The model under review builds one solid part; all positions refer to its coordinate system, in mm. Coordinates: 2 decimals unless noted, no trailing zeros. Order: outer loops, then holes, each group sorted by start corner. A loop starts at its lowest first (then second) coordinate and runs counter-clockwise, first axis right, second up. Notation, with made-up numbers: (49.25, 24) - (86.25, 24) arc R32 ccw to (86.25, 53) - close; hole circle Ø3 at (-35.75, 57). An arc over 180 degrees is marked (long way). Answer in a Markdown table with one row per item.
```python
from build123d import *

# Parameters (mm, degrees)
SKETCH1_W           = 863.6
SKETCH1_H           = 457.2
BOSS_EXTRUDE1_DEPTH = 3.175
SKETCH2_R           = 38.1
SKETCH2_R_2         = 22.225
CUT_EXTRUDE1_DEPTH  = 489.589071332


with BuildPart() as part:
    # Sketch1 → Boss-Extrude1 (new body)
    with BuildSketch(Plane.XY):
        Rectangle(SKETCH1_W, SKETCH1_H)
    extrude(amount=BOSS_EXTRUDE1_DEPTH)

    # Sketch2 → Cut-Extrude1 (cut, through all)
    with BuildSketch(Plane.XY.offset(3.175)):
        with Locations((230.738100004, 0)):
            Circle(SKETCH2_R)
        with Locations((230.738100004, -139.7)):
            Circle(SKETCH2_R)
        with Locations((179.938100004, -67.222799997)):
            Circle(SKETCH2_R_2)
        with Locations((281.538100004, -67.222799997)):
            Circle(SKETCH2_R_2)
        with Locations((179.938100004, 72.477200003)):
            Circle(SKETCH2_R_2)
        with Locations((281.538100004, 72.477200003)):
            Circle(SKETCH2_R_2)
        with Locations((-40.855899988, 120.65)):
            Circle(SKETCH2_R)
    extrude(amount=-CUT_EXTRUDE1_DEPTH, mode=Mode.SUBTRACT)


solid = part.part
```
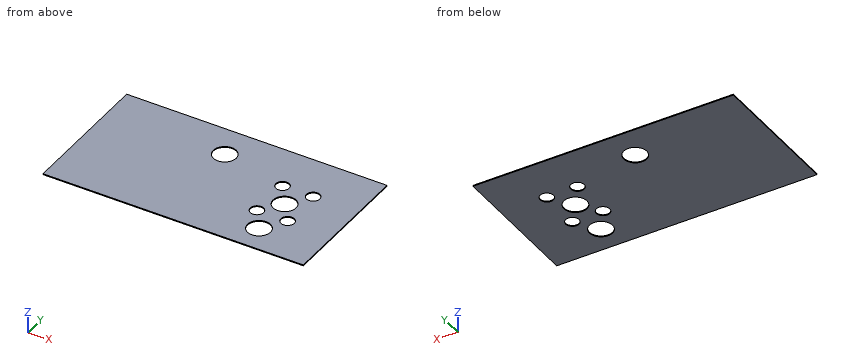
Item 1: Clearance check with a flat-ended pin moving along its axis: pin 1 Ø1.5 at (x, y) = (96, -13) entering from -Z. State where the tip first meets the part, or that it passes through.
Check values:
| item | result |
|---|---|
| pin 1 | z = 0 |
Item 2: We need section C-C, the plane z = 1.4. Write out the cut boundary in (x, y) (3 decimals), then the cut area to 3 significant figures.
Check values:
| item | result |
|---|---|
| outline | (-431.8, -228.6) - (431.8, -228.6) - (431.8, 228.6) - (-431.8, 228.6) - close; hole circle Ø76.2 at (-40.856, 120.65); hole circle Ø44.45 at (179.938, -67.223); hole circle Ø44.45 at (179.938, 72.477); hole circle Ø76.2 at (230.738, -139.7); hole circle Ø76.2 at (230.738, 0); hole circle Ø44.45 at (281.538, -67.223); hole circle Ø44.45 at (281.538, 72.477) |
| area | 375,000 mm^2 |
Item 3: We need section D-D, the plane y = 108. Write out the cut boundary in (x, z) (3 decimals).
Check values:
| item | result |
|---|---|
| outline | (-431.8, 0) - (-76.795, 0) - (-76.795, 3.175) - (-431.8, 3.175) - close; (-4.917, 0) - (431.8, 0) - (431.8, 3.175) - (-4.917, 3.175) - close |
Item 4: To check wall thickness, follow line 1 (X direction, y = -53.5, z = 1.7); line 2 (X direction, y = 92, z = 0.85); line 3 (X direction, y = 112.5, z = 0.8). State the ranges of each line that lie inside material, in increasing order. Write a range as from..to.
Check values:
| item | result |
|---|---|
| line 1 | -431.8..162.46, 197.42..264.06, 299.02..431.8 |
| line 2 | -431.8..-65.97, -15.74..169.32, 190.56..270.92, 292.16..431.8 |
| line 3 | -431.8..-78.07, -3.64..431.8 |
Item 5: We need section A-A, the plane y = -139.7. Write out the cut boundary in (x, z) (3 decimals).
Check values:
| item | result |
|---|---|
| outline | (-431.8, 0) - (192.638, 0) - (192.638, 3.175) - (-431.8, 3.175) - close; (268.838, 0) - (431.8, 0) - (431.8, 3.175) - (268.838, 3.175) - close |
Item 6: We need section B-B, the plane x = 215. Write out the cut boundary in (y, z) (3 decimals).
Check values:
| item | result |
|---|---|
| outline | (-228.6, 0) - (-174.398, 0) - (-174.398, 3.175) - (-228.6, 3.175) - close; (-105.002, 0) - (-34.698, 0) - (-34.698, 3.175) - (-105.002, 3.175) - close; (34.698, 0) - (228.6, 0) - (228.6, 3.175) - (34.698, 3.175) - close |
